```python
from build123d import *

# Parameters (mm, degrees)
PAD_DEPTH         = 0.4
POCKET_DEPTH      = 1.3027
POCKET_DEPTH_BACK = -1.724987
SKETCH002_W       = 2.5
SKETCH002_H       = 0.9
PAD001_DEPTH      = 0.5
SKETCH003_W       = 2.5
SKETCH003_H       = 0.6
POCKET001_DEPTH   = 0.3
FILLET_R          = 0.1


with BuildPart() as part:
    # Sketch → Pad (new body)
    with BuildSketch(Plane.YZ):
        with BuildLine():
            Line((-0.55, 0), (0.484315, 0))
            ThreePointArc((0.484315, 0), (0.715251, 0.073399), (0.861435, 0.266658))
            Line((0.86144, 0.266671), (0.861435, 0.266658))
            ThreePointArc((1.05, 0.4), (0.934532, 0.363301), (0.86144, 0.266671))
            Line((1.05, 0.4), (3.75, 0.4))
            ThreePointArc((3.75, 0.4), (3.798804, 0.402388), (3.847142, 0.409527))
            Line((3.847142, 0.409527), (4.828087, 0.603811))
            ThreePointArc((4.828087, 0.603811), (5.022026, 0.678974), (5.17865, 0.815833))
            ThreePointArc((7.282105, 0.706415), (6.258318, 1.298245), (5.17865, 0.815833))
            Line((7.45, 0.815094), (7.282105, 0.706415))
            ThreePointArc((7.45, 0.815094), (6.268711, 1.497974), (5.022942, 0.941351))
            ThreePointArc((4.78923, 0.8), (4.918525, 0.85011), (5.022942, 0.941351))
            Line((3.808285, 0.605716), (4.78923, 0.8))
            ThreePointArc((3.75, 0.6), (3.779282, 0.601433), (3.808285, 0.605716))
            Line((1.05, 0.6), (3.75, 0.6))
            ThreePointArc((1.05, 0.6), (0.81906, 0.526599), (0.672876, 0.333333))
            ThreePointArc((0.484311, 0.2), (0.599783, 0.2367), (0.672876, 0.333333))
            Line((0.484311, 0.2), (-0.55, 0.2))
            Line((-0.55, 0.2), (-0.55, 0))
        make_face()
    extrude(amount=PAD_DEPTH)

    # Sketch001 (on Face15 of Pad) → Pocket (cut, two sides)
    with BuildSketch(Plane(origin=(0, 0.02831, -0.142936), x_dir=(0, -0.980945, -0.194284), z_dir=(0, -0.194284, 0.980945))) as pocket_sk:
        Polygon((-3.795115, 0.4), (-4.853401, 0.3), (-7.466403, 0.3), (-7.466403, 0.4), align=None)
        Polygon((-3.795115, 0), (-4.853401, 0.1), (-7.466403, 0.1), (-7.466403, 0), align=None)
    extrude(amount=-POCKET_DEPTH, mode=Mode.SUBTRACT)
    extrude(pocket_sk.sketch, amount=-POCKET_DEPTH_BACK, mode=Mode.SUBTRACT)

    # Sketch002 (on Face14 of Pocket) → Pad001 (join)
    with BuildSketch(Plane(origin=(0, 0, 0.6), x_dir=(0, -1, 0), z_dir=(0, 0, 1))):
        with Locations((-2.3, 0.2)):
            Rectangle(SKETCH002_W, SKETCH002_H)
    extrude(amount=-PAD001_DEPTH)

    # Sketch003 (on Face16 of Pad001) → Pocket001 (cut)
    with BuildSketch(Plane.YX.offset(-0.1)):
        with Locations((2.3, 0.2)):
            Rectangle(SKETCH003_W, SKETCH003_H)
    extrude(amount=-POCKET001_DEPTH, mode=Mode.SUBTRACT)

    # Fillet
    fillet_edges = [part.edges().sort_by_distance(p)[0] for p in [
        (0.65, 2.3, 0.6),
        (-0.25, 2.3, 0.6),
    ]]
    fillet(fillet_edges, radius=FILLET_R)


with BuildPart() as part_1:
    # Body placement: moved
    add(part.part.moved(Location((-0.2, 0, 0))))


solid = part_1.part
```
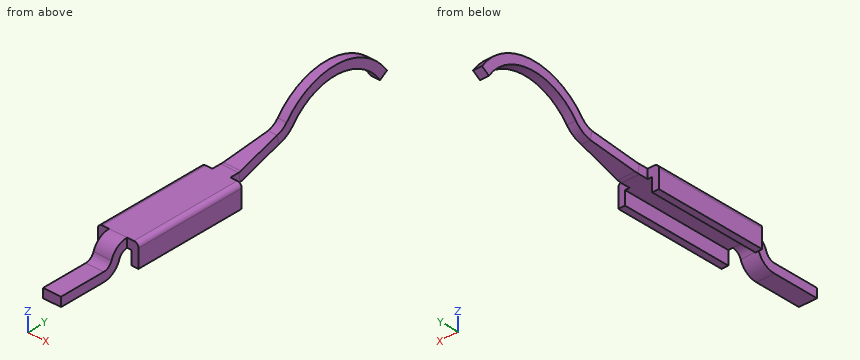
For this review, take the finished solid that the model builds, in its own axes (mm). Round coordinates to 2 decimals unless told otherwise and drop trailing zeros. Loops run counter-clockwise (first coordinate to the right, second up) from the corner with the lowest first, then second, coordinate; pieces in that order, holes last.
Q1. Add section C-C on y = 4.5. Write out the cut boundary in (x, z).
Result sheet:
outline: (-0.13, 0.54) - (0.13, 0.54) - (0.13, 0.74) - (-0.13, 0.74) - close
Q2. Insertion check: pin 1 Ø0.7 at (y, z) = (0.5, 0.5) entering from +X. The pin has a flat end and moves straight along its axis. Give the tip position at first contact, or say it passes through.
Result sheet:
pin 1: stops at x = 0.2
Q3. Add section B-B on z = 1.1. Write out the cut boundary in (x, y).
Result sheet:
outline: (-0.1, 5.17) - (0.1, 5.17) - (0.1, 5.5) - (-0.1, 5.5) - close; (-0.1, 6.88) - (0.1, 6.88) - (0.1, 7.21) - (-0.1, 7.21) - close
Q4. Add section A-A on y = 3. Write out the cut boundary in (x, z), plus the area to 3 significant figures.
Result sheet:
outline: (-0.45, 0.1) - (-0.3, 0.1) - (-0.3, 0.4) - (0.3, 0.4) - (0.3, 0.1) - (0.45, 0.1) - (0.45, 0.5) arc R0.1 ccw to (0.35, 0.6) - (-0.35, 0.6) arc R0.1 ccw to (-0.45, 0.5) - close
area: 0.266 mm2
Q5. To check wall thickness, follow line 1 along Z through (x, y) = (0.05, 3.75); line 2 along Z through (x, y) = (-0.05, 0.25); line 3 along X through (y, z) = (6.75, 1.3). State the ranges of each line that lie inside material, in increasing order.
Result sheet:
line 1: z = 0.4 to 0.6
line 2: z = 0 to 0.2
line 3: x = -0.1 to 0.1
